Autodesk Inventor part; units mm, degrees
ref_plane "Work Plane4" through (9.1457, 13.7679, 19.8187) normal (0, -1, 0) x (-1, 0, 0)
ref_plane "Work Plane5" through (1.2414, 11.6271, 11.9106) normal (0, 1, 0) x (0, 0, 1)
ref_plane "YZ Plane" through (0, 0, 0) normal (1, 0, 0) x (0, 1, 0)
ref_plane "Work Plane1" through (9.1457, 10.0679, 19.8187) normal (0, 1, 0) x (-1, 0, 0)
sketch "Sketch1" plane through (9.1457, 10.0679, 19.8187) normal (0, 1, 0) x (-1, 0, 0)
  circle A0 centre (-8, -17.9) radius 2 construction
  circle A1 centre (-8, 17.9) radius 2 construction
  arc A2 (7.7389, -5.1575) -> (7.7389, 5.1575) centre (0, 0) ccw
  arc A3 (-4.4444, 19.7325) -> (-11.2421, 15.5572) centre (-8, 17.9) ccw
  line L0 (-7.847, 10.8589) -> (-11.2421, 15.5572)
  arc A4 (-7.7389, 5.1575) -> (-7.847, 10.8589) centre (-11.8996, 7.9303) ccw
  arc A5 (-7.847, -10.8589) -> (-7.7389, -5.1575) centre (-11.8996, -7.9303) ccw
  line L1 (-11.2421, -15.5572) -> (-7.847, -10.8589)
  arc A6 (-11.2421, -15.5572) -> (-4.4444, -19.7325) centre (-8, -17.9) ccw
  circle A7 centre (0, 0) radius 7.3 construction
  circle A8 centre (0, 0) radius 5 construction
  circle A9 centre (0, 0) radius 2.5 construction
  circle A10 centre (-8, 17.9) radius 2.3
  circle A11 centre (-8, -17.9) radius 2.3
  circle A12 centre (8, -17.9) radius 2 construction
  circle A13 centre (8, 17.9) radius 2 construction
  arc A14 (4.4444, -19.7325) -> (-4.4444, -19.7325) centre (0, -22.0231) ccw
  arc A15 (4.4444, -19.7325) -> (11.2421, -15.5572) centre (8, -17.9) ccw
  line L2 (11.2421, -15.5572) -> (7.847, -10.8589)
  arc A16 (7.7389, -5.1575) -> (7.847, -10.8589) centre (11.8996, -7.9303) ccw
  arc A17 (7.847, 10.8589) -> (7.7389, 5.1575) centre (11.8996, 7.9303) ccw
  line L3 (7.847, 10.8589) -> (11.2421, 15.5572)
  arc A18 (11.2421, 15.5572) -> (4.4444, 19.7325) centre (8, 17.9) ccw
  arc A19 (-4.4444, 19.7325) -> (4.4444, 19.7325) centre (0, 22.0231) ccw
  circle A20 centre (8, -17.9) radius 2.3
  circle A21 centre (8, 17.9) radius 2.3
  arc A22 (1.8, 2.1448) -> (-1.8, 2.1448) centre (0, 0) ccw construction
  line L4 (-1.8, -2.1448) -> (-1.8, 2.1448) construction
  arc A23 (-1.8, -2.1448) -> (1.8, -2.1448) centre (0, 0) ccw construction
  line L5 (1.8, 2.1448) -> (1.8, -2.1448) construction
  line L6 (1.5, 2) -> (1.5, -2)
  arc A24 (-1.5, -2) -> (1.5, -2) centre (0, 0) ccw
  line L7 (-1.5, -2) -> (-1.5, 2)
  arc A25 (1.5, 2) -> (-1.5, 2) centre (0, 0) ccw
  circle A26 centre (0, 0) radius 2.8
  arc A27 (-7.7389, 5.1575) -> (-7.7389, -5.1575) centre (0, 0) ccw
  point P0 (9.1457, -19.8187)
  point P1 (-13.1394, 9.646)
  point P2 (-13.1394, -9.646)
  point P3 (13.1394, -9.646)
  point P4 (13.1394, 9.646)
  point P5 (-11.8996, 7.9303)
  point P6 (-11.8996, -7.9303)
  point P7 (11.8996, -7.9303)
  point P8 (11.8996, 7.9303)
  point P9 (11.8996, -7.9303)
  point P10 (11.8996, 7.9303)
  point P11 (-11.8996, 7.9303)
  point P12 (-11.8996, -7.9303)
  point P13 (11.8996, -7.9303)
  point P14 (11.8996, 7.9303)
  point P15 (0, 0)
  point P16 (11.8996, -7.9303)
  point P17 (11.8996, 7.9303)
  point P18 (11.8996, -7.9303)
  point P19 (11.8996, 7.9303)
  point P20 (-11.8996, 7.9303)
  point P21 (-11.8996, -7.9303)
  dimension "d1" = 0.3
  dimension "d2" = 0.3
  dimension "d8" = 0.3
  dimension "d9" = 0.3
  dimension "d20" = 0.3
ref_plane "Work Plane2" through (17.1457, 15.7679, 19.8187) normal (0, -1, 0) x (-1, 0, 0)
extrude "Extrusion1" add sketch "Sketch1" along normal up to surface (5.7 mm away) contours A16 L2 A15 A14 A6 L1 A5 A27 A4 L0 A3 A19 A18 L3 A17 A2
sketch "Sketch3" plane through (9.1457, 15.7679, 41.8418) normal (0, 1, 0) x (1, 0, 0)
  circle A0 centre (0, 22.0231) radius 5 construction
  circle A1 centre (0, 22.0231) radius 5.3
  point P0 (-9.1457, 41.8418)
  dimension "d11" = 0.3
ref_plane "Work Plane4" through (9.1457, 13.7679, 19.8187) normal (0, -1, 0) x (-1, 0, 0)
extrude "Extrusion3" cut sketch "Sketch3" against normal up to surface (2 mm away)
sketch "Sketch4" plane through (9.1457, 13.7679, 19.8187) normal (0, 1, 0) x (1, 0, 0)
  circle A0 centre (0, 0) radius 3.8
  circle A1 centre (0, 0) radius 5.3
  point P0 (-9.1457, 19.8187)
extrude "Extrusion4" cut sketch "Sketch4" against normal blind 0.1
ref_plane "Work Plane5" through (1.2414, 11.6271, 11.9106) normal (0, 1, 0) x (0, 0, 1)
properties part number "shaft encap lid"
Design review of the part built by this model. Coordinates are the model's own, in mm. A direction names the side the tool comes from. Give positions to 0.01 mm unless a question says otherwise; leave off trailing zeros. Order: outer loops, then holes, each group sorted by start corner. A loop starts at its lowest first (then second) coordinate and runs counter-clockwise, first axis right, second up. Notation, with made-up numbers: M 25.25,12.25 L 69.25,12.25 A27 cw 69.25,50.25 Z; hole C -36,-0.75 d8. An arc over 180 degrees is marked long. One line per question, with ' | ' between items. Start each with the question number.
Q1. Machinability: for faces 1 (the face through (4.94, 14.733, 23.044)), 2 (the face through (-1.03, 12.88, -1.44)), 3 (the face through (18.666, 12.878, 32.994)), 4 (the face through (-0.375, 12.878, 32.994)), which of the approach directions +Z, -Z, +X, -X, +Y, -Y give a long, thin tool a straight path to every point of the face, cutting with its end or side? Answer none if there is none.
Q2. We need section D-D (y = 14.6). Write out the cut boundary in (x, z), plus the area to 3 significant figures.
Q3. The part is to be moulded in two halves that separate along X. For faces 5 (the face through (9, 10.068, 25)), 6 (the face through (2.244, 12.878, 11.751)), 7 (the face through (19.317, 12.878, 41.078)), say which applies: +X half, -X half, draft (parallel to the pull), parting line (faces both ways), or undercut.
Q4. We need section B-B (y = 11.4). Write out the cut boundary in (x, z).
Q5. For L1, parallel to Z at x = 19.25, y = 12.65; L2, parallel to X at y = 10.8, z = 2; L3, parallel to Z at x = 15.5, y = 11.55, list the stretches that pass through material, from the lowest coordinate up. Write a range as [from, to].
Q6. We need section C-C (z = 21.5). Write out the cut boundary in (x, y).
Q7. For pin 1 Ø6.5 at (x, z) = (9.15, 19.82) entering from -Y; pin 2 Ø1 at (x, y) = (12, 12) entering from -Z; pin 3 Ø3 at (x, z) = (1.15, 37.72) entering from +Y; pin 4 Ø1.5 at (x, y) = (5, 13.5) entering from +Z, all flat-tipped, find the tip position at first contact; note any pin that passes through.
Q8. We need section A-A (x = 10.25). Write out the cut boundary in (y, z).
Returned:
1) face 1: +Y | face 2: +Y, -Y | face 3: +X, +Y, -Y | face 4: -X, +Y, -Y
2) outline: M -2.1,4.26 A4 ccw long 4.7,0.09 A5 cw 13.59,0.09 A4 ccw long 20.39,4.26 L 16.99,8.96 A5 cw 16.88,14.66 A9.3 ccw 16.88,24.98 A5 cw 16.99,30.68 L 20.39,35.38 A4 ccw long 13.59,39.55 A5 cw 4.7,39.55 A4 ccw long -2.1,35.38 L 1.3,30.68 A5 cw 1.41,24.98 A9.3 ccw 1.41,14.66 A5 cw 1.3,8.96 Z; hole C 1.15,1.92 d4.6; hole C 1.15,37.72 d4.6; hole C 9.15,19.82 d10.6; hole C 17.15,1.92 d4.6; hole C 17.15,37.72 d4.6 | area: 577 mm2
3) face 5: draft | face 6: -X half | face 7: undercut
4) outline: M -2.1,4.26 A4 ccw long 4.7,0.09 A5 cw 13.59,0.09 A4 ccw long 20.39,4.26 L 16.99,8.96 A5 cw 16.88,14.66 A9.3 ccw 16.88,24.98 A5 cw 16.99,30.68 L 20.39,35.38 A4 ccw long 13.59,39.55 A5 cw 4.7,39.55 A4 ccw long -2.1,35.38 L 1.3,30.68 A5 cw 1.41,24.98 A9.3 ccw 1.41,14.66 A5 cw 1.3,8.96 Z; hole C 1.15,1.92 d4.6; hole C 1.15,37.72 d4.6; hole C 9.15,19.82 d5.6; hole C 17.15,1.92 d4.6; hole C 17.15,37.72 d4.6
5) L1: [-1.48, 0.99], [2.85, 5.84], [33.8, 36.79], [38.65, 41.12] | L2: [-2.85, -1.15], [3.44, 6.44], [11.85, 14.85], [19.44, 21.14] | L3: [-1.73, 0.31], [3.53, 36.11], [39.33, 41.36]
6) outline: M 0,10.07 L 6.91,10.07 L 6.91,13.77 L 5.74,13.77 L 5.74,13.67 L 4.12,13.67 L 4.12,15.77 L 0,15.77 Z; M 11.38,10.07 L 18.29,10.07 L 18.29,15.77 L 14.17,15.77 L 14.17,13.67 L 12.55,13.67 L 12.55,13.77 L 11.38,13.77 Z
7) pin 1: y = 10.07 | pin 2: z = 1.5 | pin 3: through | pin 4: z = 40.24
8) outline: M 10.07,2.67 L 15.77,2.67 L 15.77,14.64 L 13.67,14.64 L 13.67,16.18 L 13.77,16.18 L 13.77,17.25 L 10.07,17.25 Z; M 10.07,22.39 L 13.77,22.39 L 13.77,23.45 L 13.67,23.45 L 13.67,25 L 15.77,25 L 15.77,36.97 L 10.07,36.97 Z
